The listing builds one solid part. Answer for the finished solid, in the listing's coordinates (mm). Face numbers are marked on the shaded views. A direction names the side the tool comes from. Give positions to 0.01 mm unless a question says otherwise; leave off trailing zeros. Order: outer loops, then holes, each group sorted by start corner. A loop starts at its lowest first (then second) coordinate and runs counter-clockwise, first axis right, second up. Notation, with made-up numbers: (-37, -33) - (-7, -33) arc R23 cw to (-7, -24) - close; hole circle Ø8 at (11.5, -17.75). An arc over 180 degrees is marked (long way). Answer in a Markdown table with one row per item. Add a question column.
```python
from build123d import *

# Parameters (mm, degrees)
CROQUIS1_R              = 7.5
SALIENTE_EXTRUIR1_DEPTH = 21
CROQUIS2_R              = 1
CORTAR_EXTRUIR1_DEPTH   = 10.5
CROQUIS3_W              = 6
CROQUIS3_H              = 18
CORTAR_EXTRUIR2_DEPTH   = 6
REDONDEO1_R             = 4


with BuildPart() as part:
    # Croquis1 → Saliente-Extruir1 (new body)
    with BuildSketch(Plane.XY):
        Circle(CROQUIS1_R)
    extrude(amount=SALIENTE_EXTRUIR1_DEPTH)

    # Croquis2 → Cortar-Extruir1 (cut, symmetric)
    with BuildSketch(Plane(origin=(0, 0, 0), x_dir=(0, 0, -1), z_dir=(1, 0, 0))):
        with Locations((-18, 0)):
            Circle(CROQUIS2_R)
    extrude(amount=CORTAR_EXTRUIR1_DEPTH, both=True, mode=Mode.SUBTRACT)

    # Croquis3 → Cortar-Extruir2 (cut)
    with BuildSketch(Plane.XY.offset(21)):
        Rectangle(CROQUIS3_W, CROQUIS3_H)
    extrude(amount=-CORTAR_EXTRUIR2_DEPTH, mode=Mode.SUBTRACT)

    # Redondeo1
    redondeo1_edges = [part.edges().sort_by_distance(p)[0] for p in [
        (-7.5, 0, 0),
    ]]
    fillet(redondeo1_edges, radius=REDONDEO1_R)


solid = part.part
```
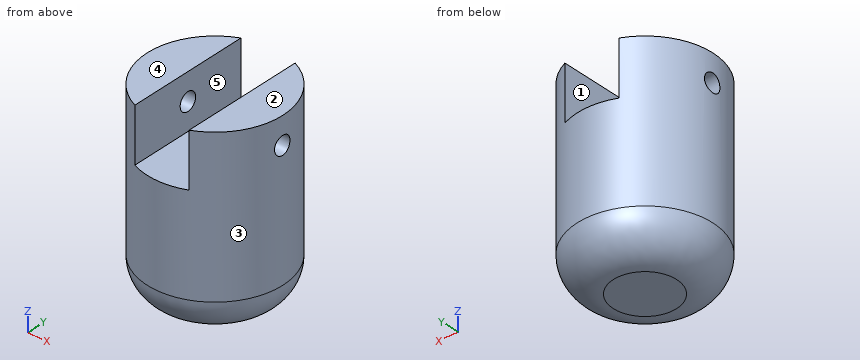
(1) Each of these flat-tipped pins is pushed along its axis until it touches: P1, Ø3, axis at x = -5.5, z = 12, coming from the +Y side; P2, Ø2, axis at x = 1.5, z = 8.5, coming from the +Y side; P3, Ø1.5, axis at y = 1, z = 16.5, coming from the +X side; P4, Ø8, axis at x = -5.5, y = -3.5, coming from the -Z side. Where does it stop, or does it pass through?
(2) Find section A-A, the plane z = 18. Write down the section's boundary in (x, y), plus the area to 3 significant figures.
(3) For the marked faces 1 and 2, determine the directions among +Z, -Z, +X, -X, +Y, -Y from which every point of the face is accessible in a straight line to the end or side of a thin tool.
(4) The mould has two halves that part along X. Classify the marked faces 3, 4 and 5: +X half, -X half, draft (parallel to the pull), parting line (faces both ways), or undercut.
(5) Find section C-C, the plane z = 7.25. Write down the section's boundary in (x, y), plus the area to 3 significant figures.
(6) Find section B-B, the plane y = 0. Give the number of separate pieces and of enclosed holes in the cut face, plus the area to 3 significant figures.
(7) Straight lines are drawn through the part: line 1 (X direction, y = -3.75, z = 19.5); line 2 (Y direction, x = 4, z = 18); line 3 (Z direction, x = 6.1, y = 0). For each, find the intervals that lie inside material, in ascending order.
Answer key:
| question | item | result |
|---|---|---|
| 1 | P1 | y = 6.34 |
| 1 | P2 | y = 7.48 |
| 1 | P3 | x = 7.5 |
| 1 | P4 | z = 0 |
| 2 | outline | (-7.43, -1) arc R7.5 ccw to (-3, -6.87) - (-3, -1) - close; (-7.43, 1) - (-3, 1) - (-3, 6.87) arc R7.5 ccw to start; (3, -6.87) arc R7.5 ccw to (7.43, -1) - (3, -1) - close; (3, 1) - (7.43, 1) arc R7.5 ccw to (3, 6.87) - close |
| 2 | area | 71.3 mm² |
| 3 | face 1 | +Z, +Y, -Y |
| 3 | face 2 | +Z, +X, -X, +Y, -Y |
| 4 | face 3 | parting line |
| 4 | face 4 | draft |
| 4 | face 5 | undercut |
| 5 | outline | circle Ø15 at (0, 0) |
| 5 | area | 177 mm² |
| 6 | separate pieces | 3 |
| 6 | enclosed holes | 0 |
| 6 | area | 254 mm² |
| 7 | line 1 | -6.5 to -3, 3 to 6.5 |
| 7 | line 2 | -6.34 to -1, 1 to 6.34 |
| 7 | line 3 | 0.96 to 17, 19 to 21 |
